from build123d import *

# Parameters (mm, degrees)
SKETCH1_W           = 90
SKETCH1_H           = 66
BOSS_EXTRUDE1_DEPTH = 76
SKETCH2_W           = 90
SKETCH2_H           = 36
CUT_EXTRUDE1_DEPTH  = 66
SKETCH3_W           = 90
SKETCH3_H           = 76
BOSS_EXTRUDE4_DEPTH = 5
SKETCH11_W          = 90
SKETCH11_H          = 76
BOSS_EXTRUDE5_DEPTH = 5
SKETCH12_W          = 80
SKETCH12_H          = 71
CUT_EXTRUDE9_DEPTH  = 15
SKETCH13_W          = 80
SKETCH13_H          = 71
CUT_EXTRUDE10_DEPTH = 15
SKETCH14_R          = 2.5
CUT_EXTRUDE11_DEPTH = 5
SKETCH15_R          = 2.5
CUT_EXTRUDE12_DEPTH = 5
FILLET1_R           = 10
FILLET2_R           = 5


with BuildPart() as part:
    # Sketch1 → Boss-Extrude1 (new body)
    with BuildSketch(Plane(origin=(0, 0, 0), x_dir=(1, 0, 0), z_dir=(0, 1, 0))):
        Rectangle(SKETCH1_W, SKETCH1_H)
    extrude(amount=BOSS_EXTRUDE1_DEPTH)

    # Sketch2 → Cut-Extrude1 (cut)
    with BuildSketch(Plane(origin=(0, 76, 0), x_dir=(1, 0, 0), z_dir=(0, 1, 0))):
        Rectangle(SKETCH2_W, SKETCH2_H)
    extrude(amount=-CUT_EXTRUDE1_DEPTH, mode=Mode.SUBTRACT)

    # Sketch3 → Boss-Extrude4 (add)
    with BuildSketch(Plane(origin=(0, 0, -33), x_dir=(-1, 0, 0), z_dir=(0, 0, -1))):
        with Locations((0, 38)):
            Rectangle(SKETCH3_W, SKETCH3_H)
    extrude(amount=BOSS_EXTRUDE4_DEPTH)

    # Sketch11 → Boss-Extrude5 (add)
    with BuildSketch(Plane.XY.offset(33)):
        with Locations((0, 38)):
            Rectangle(SKETCH11_W, SKETCH11_H)
    extrude(amount=BOSS_EXTRUDE5_DEPTH)

    # Sketch12 → Cut-Extrude9 (cut)
    with BuildSketch(Plane.XY.offset(38)):
        with Locations((0, 35.5)):
            Rectangle(SKETCH12_W, SKETCH12_H)
    extrude(amount=-CUT_EXTRUDE9_DEPTH, mode=Mode.SUBTRACT)

    # Sketch13 → Cut-Extrude10 (cut)
    with BuildSketch(Plane(origin=(0, 0, -38), x_dir=(-1, 0, 0), z_dir=(0, 0, -1))):
        with Locations((0, 35.5)):
            Rectangle(SKETCH13_W, SKETCH13_H)
    extrude(amount=-CUT_EXTRUDE10_DEPTH, mode=Mode.SUBTRACT)

    # Sketch14 → Cut-Extrude11 (cut)
    with BuildSketch(Plane(origin=(0, 76, 0), x_dir=(1, 0, 0), z_dir=(0, 1, 0))):
        with Locations(Location((0, 27.5, 0), (0, 0, 270))):
            Circle(SKETCH14_R)
    extrude(amount=-CUT_EXTRUDE11_DEPTH, mode=Mode.SUBTRACT)

    # Sketch15 → Cut-Extrude12 (cut)
    with BuildSketch(Plane(origin=(0, 76, 0), x_dir=(1, 0, 0), z_dir=(0, 1, 0))):
        with Locations(Location((0, -27.5, 0), (0, 0, 270))):
            Circle(SKETCH15_R)
    extrude(amount=-CUT_EXTRUDE12_DEPTH, mode=Mode.SUBTRACT)

    # Fillet1
    fillet1_edges = [part.edges().sort_by_distance(p)[0] for p in [
        (-45, 38, -38),
        (45, 38, -38),
        (-45, 38, 38),
        (45, 38, 38),
    ]]
    fillet(fillet1_edges, radius=FILLET1_R)

    # Fillet2
    fillet2_edges = [part.edges().sort_by_distance(p)[0] for p in [
        (45, 76, -23),
        (42.071067812, 76, -35.071067812),
        (-42.071067812, 76, -35.071067812),
        (45, 76, 23),
        (42.071067812, 76, 35.071067812),
        (0, 76, 38),
        (-42.071067812, 76, 35.071067812),
        (0, 76, -38),
        (-45, 76, -23),
        (-45, 76, 23),
    ]]
    fillet(fillet2_edges, radius=FILLET2_R - 0.0001)  # a hair under: the kernel refuses the full size


solid = part.part
Design review of the part built by this model. Coordinates are the model's own, in mm. A direction names the side the tool comes from. Coordinates: 2 decimals unless noted, no trailing zeros. Order: outer loops, then holes, each group sorted by start corner. A loop starts at its lowest first (then second) coordinate and runs counter-clockwise, first axis right, second up. Notation, with made-up numbers: (-39, -20) -> (16, -20) arc R16 ccw to (16, 5) -> close; hole circle Ø2 at (10, 80). An arc over 180 degrees is marked (long way). Use one line per item in the form item = value. Start each with the question number.
(1) The part is to be moulded in two halves that separate along Z. For faces 5 (the flat face through (-1, 43, 18)), 6 (the cylindrical face through (0, 74, 25)), 7 (the flat face through (-45, 35, -19)), 8 (the cylindrical face through (-44.109, 35.997, -32.126)), say which applies: +Z half, -Z half, draft (parallel to the pull), parting line (faces both ways), or undercut.
(2) For faces 1 (the flat face through (-1, 71, 31)), 2 (the flat face through (-1, 76, 24)), 3 (the flat face through (-1, 10, 0)), 4 (the flat face through (40, 35, -30)), list the 3-axis set-ups (+Z, -Z, +X, -X, +Y, -Y) from which the entire face can be reached by the end or side of a thin tool; tool diameter is ignored.
(3) Insertion check: pin 1 (20 mm diameter, centred on x = -15.5, y = 31, fed in from -Z); pin 2 (1.5 mm diameter, centred on x = 23.5, y = 35, fed in from +Z); pin 3 (7 mm diameter, centred on y = 44, z = -33, fed in from +X). Each pin has a flat end and moves straight along its axis. Give the tip position at first contact, or say it passes through.
(4) For probe 1 along Z at (x, y) = (-1.5, 46); probe 2 along X at (y, z) = (52, 28); probe 3 along Y at (x, z) = (22.5, -0.5), list the stretches that pass through material, from the lowest coordinate up.
(5) Add section B-B on y = 68. State the section outline as (x, z) points.
(6) Add section D-D on z = 10. State the section outline as (x, y) points, plus the area to 3 significant figures.
(7) Add section A-A on x = 0. Give the number of separate pieces and of enclosed holes in the cut face, plus the area to 3 significant figures.
Answer block:
q1.face_5 = undercut
q1.face_6 = undercut
q1.face_7 = draft
q1.face_8 = -Z half
q2.face_1 = +Z, -Y
q2.face_2 = +Z, -Z, +X, -X, +Y
q2.face_3 = +X, -X, +Y
q2.face_4 = -Z, -Y
q3.pin_1 = -23
q3.pin_2 = 23
q3.pin_3 = 44.89
q4.probe_1 = -23 to -18, 18 to 23
q4.probe_2 = -45 to -40, 40 to 45
q4.probe_3 = 0 to 10
q5.outline = (-45, -28) arc R10 ccw to (-40, -36.66) -> (-40, -23) -> (40, -23) -> (40, -36.66) arc R10 ccw to (45, -28) -> (45, -18) -> (-45, -18) -> close; (-45, 18) -> (45, 18) -> (45, 28) arc R10 ccw to (40, 36.66) -> (40, 23) -> (-40, 23) -> (-40, 36.66) arc R10 ccw to (-45, 28) -> close
q6.outline = (-45, 0) -> (45, 0) -> (45, 10) -> (-45, 10) -> close
q6.area = 900 mm²
q7.separate_pieces = 3
q7.enclosed_holes = 0
q7.area = 1,210 mm²
